Build history of the part. All positions in model axes, mm. Face numbers are marked on the shaded views. A direction names the side the tool comes from. Give positions to 0.01 mm unless a question says otherwise; leave off trailing zeros. Loops run counter-clockwise (first coordinate to the right, second up) from the corner with the lowest first, then second, coordinate; pieces in that order, holes last. Notation, with made-up numbers: (48, -26.5) -> (52, -26.5) arc R21 cw to (52, -17.5) -> close; hole circle Ø3 at (4.5, 80.25). An arc over 180 degrees is marked (long way). Answer as a JSON object with one key per item and string values. Group by question number.
Q1. Band-saw the part on A-A, the plane x = 0. Write the cut outline in (y, z), plus the area to 3 significant figures.
Q2. Drop flat-ended pins along their axis: pin 1 (2 mm diameter, centred on y = -5, z = 47.5, fed in from -X); pin 2 (2 mm diameter, centred on x = 4.5, z = 37, fed in from +Y); pin 3 (6 mm diameter, centred on y = -3.5, z = 34, fed in from -X). Give the stop position or say it passes through.
Q3. Wall check: probe 1 along Z at (x, y) = (14, 14); probe 2 along Z at (x, y) = (20, 15); probe 3 along X at (y, z) = (-3, 19.5). Give the ranges that are in metal, low to high. Write a range as from..to.
Q4. Tool access for the marked faces 1 and 2: list every direction of +Z, -Z, +X, -X, +Y, -Y with a clear straight run to the whole face (end or side of a thin tool).
Q5. Band-saw the part on C-C, the plane z = 66. Write the cut outline in (x, y), plus the area to 3 significant figures.
Q6. Band-saw the part on D-D, the plane y = 23. Write the cut outline in (x, z), plus the area to 3 significant figures.
from build123d import *

# Parameters (mm, degrees)
F0_W     = 80.297806
F0_H     = 80.297806
F1_DEPTH = 12.7
F2_R     = 21.68697
F3_DEPTH = 19.05
F4_R     = 12.981603
F5_DEPTH = 25.4
F6_R     = 8.559501
F7_DEPTH = 19.05


with BuildPart() as f1:
    # F0 (on Top) → F1 (new body)
    with BuildSketch(Plane.XY):
        Rectangle(F0_W, F0_H)
    extrude(amount=F1_DEPTH)

    # F2 (on face) → F3 (join)
    with BuildSketch(Plane.XY.offset(12.7)):
        Circle(F2_R)
    extrude(amount=F3_DEPTH)

    # F4 (on face) → F5 (join)
    with BuildSketch(Plane.XY.offset(31.75)):
        Circle(F4_R)
    extrude(amount=F5_DEPTH)

    # F6 (on face) → F7 (join)
    with BuildSketch(Plane.XY.offset(57.15)):
        Circle(F6_R)
    extrude(amount=F7_DEPTH)


solid = f1.part
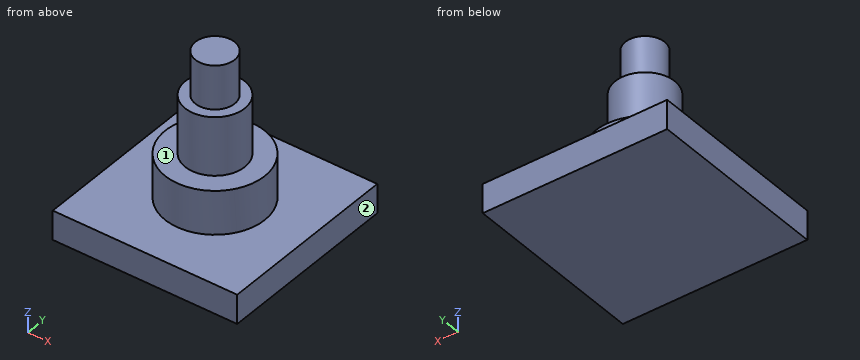
Worked answers:
{
 "1": {"outline": "(-40.15, 0) -> (40.15, 0) -> (40.15, 12.7) -> (21.69, 12.7) -> (21.69, 31.75) -> (12.98, 31.75) -> (12.98, 57.15) -> (8.56, 57.15) -> (8.56, 76.2) -> (-8.56, 76.2) -> (-8.56, 57.15) -> (-12.98, 57.15) -> (-12.98, 31.75) -> (-21.69, 31.75) -> (-21.69, 12.7) -> (-40.15, 12.7) -> close", "area": "2,830 mm2"},
 "2": {"pin 1": "x = -12.35", "pin 2": "y = 12.5", "pin 3": "x = -21.63"},
 "3": {"probe 1": "0..31.75", "probe 2": "0..12.7", "probe 3": "-21.48..21.48"},
 "4": {"face 1": "+Z", "face 2": "+Z, -Z, +X, +Y, -Y"},
 "5": {"outline": "circle Ø17.12 at (0, 0)", "area": "230 mm2"},
 "6": {"outline": "(-40.15, 0) -> (40.15, 0) -> (40.15, 12.7) -> (-40.15, 12.7) -> close", "area": "1,020 mm2"}
}
